```python
from build123d import *

# Parameters (mm, degrees)
SKETCH_2_R          = 32
EXTRUDE_2_DEPTH     = 1
SKETCH_3_R          = 32
EXTRUDE_3_DEPTH     = 28
EXTRUDE_3_TAPER     = 45
SKETCH_5_R          = 30
CUT_EXTRUDE_1_DEPTH = 1
SKETCH_6_R          = 30
CUT_EXTRUDE_2_DEPTH = 28
CUT_EXTRUDE_2_DRAFT = -45
SKETCH_7_R          = 4
EXTRUDE_5_DEPTH     = 6
EXTRUDE_5_TAPER     = 10
SKETCH_10_R         = 2
CUT_EXTRUDE_3_DEPTH = 54.749418721


with BuildPart() as part:
    # 草图2 → 凸台-拉伸2 (new body)
    with BuildSketch(Plane(origin=(0, 0, 0), x_dir=(1, 0, 0), z_dir=(0, 1, 0))):
        with Locations(Location((0, 0, 0), (0, 0, 270))):
            Circle(SKETCH_2_R)
    extrude(amount=EXTRUDE_2_DEPTH)

    # 草图3 → 凸台-拉伸3 (add)
    with BuildSketch(Plane(origin=(0, 1, 0), x_dir=(1, 0, 0), z_dir=(0, 1, 0))):
        with Locations(Location((0, 0, 0), (0, 0, 270))):
            Circle(SKETCH_3_R)
    extrude(amount=EXTRUDE_3_DEPTH, taper=EXTRUDE_3_TAPER)

    # 草图5 → 切除-拉伸1 (cut)
    with BuildSketch(Plane(origin=(0, 0, 0), x_dir=(-1, 0, 0), z_dir=(0, -1, 0))):
        with Locations(Location((0, 0, 0), (0, 0, 90))):
            Circle(SKETCH_5_R)
    extrude(amount=-CUT_EXTRUDE_1_DEPTH, mode=Mode.SUBTRACT)


with BuildPart() as cut_extrude_2_tool:
    # 草图6 → 切除-拉伸2 (with draft: the straight prism first)
    with BuildSketch(Plane(origin=(0, 1, 0), x_dir=(-1, 0, 0), z_dir=(0, -1, 0))):
        with Locations(Location((0, 0, 0), (0, 0, 90))):
            Circle(SKETCH_6_R)
    extrude(amount=-CUT_EXTRUDE_2_DEPTH)
    # 切除-拉伸2: the draft: its side faces are tilted about the plane it starts from
    cut_extrude_2_sides = [cut_extrude_2_tool.faces().sort_by_distance(p)[0] for p in [
        (0, 15, 30),
    ]]
    draft(cut_extrude_2_sides, Plane(origin=(0, 1, 0), x_dir=(-1, 0, 0), z_dir=(0, -1, 0)), CUT_EXTRUDE_2_DRAFT)


with BuildPart() as part_1:
    add(part.part)

    # 切除-拉伸2: cut by cut_extrude_2_tool
    add(cut_extrude_2_tool.part, mode=Mode.SUBTRACT)

    # 草图7 → 凸台-拉伸5 (add)
    with BuildSketch(Plane(origin=(0, 29, 0), x_dir=(1, 0, 0), z_dir=(0, 1, 0))):
        Circle(SKETCH_7_R)
    extrude(amount=EXTRUDE_5_DEPTH, taper=EXTRUDE_5_TAPER)

    # 草图10 → 切除-拉伸3 (cut, through all)
    with BuildSketch(Plane(origin=(0, 29, 0), x_dir=(-1, 0, 0), z_dir=(0, -1, 0))):
        with Locations(Location((0, 0, 0), (0, 0, 90))):
            Circle(SKETCH_10_R)
    extrude(amount=-CUT_EXTRUDE_3_DEPTH, mode=Mode.SUBTRACT)


solid = part_1.part
```
Design review of the part built by this model. Coordinates are the model's own, in mm. A direction names the side the tool comes from. Coordinates: 2 decimals unless noted, no trailing zeros. Order: outer loops, then holes, each group sorted by start corner. A loop starts at its lowest first (then second) coordinate and runs counter-clockwise, first axis right, second up. Notation, with made-up numbers: M 75.25,-37 L 119.25,-37 A20 ccw 119.25,-16 Z; hole C 56,80 d5. An arc over 180 degrees is marked long. Answer as a JSON object with one key per item and string values. Group by question number.
1) Mouldability with a two-part tool opening along Z and no side actions: class faces 3 (the conical face through (2.54, 24.53, 8.08)), 4 (the flat face through (1, 35, 2)), 5 (the conical face through (-6.699, 24.137, 1.488)) as pulls with the +Z half, pulls with the -Z half, needs draft (parallel to the pull), parting line crosses it, or undercut.
2) Tool access review of faces 1 (the cylindrical face through (1.32, 0.49, 29.97)), 2 (the conical face through (-0.436, 32.709, -3.318)): name each direction out of +Z, -Z, +X, -X, +Y, -Y from which nothing blocks a thin tool from reaching the whole face with its end or side.
3) Wall thickness on L1, parallel to X at y = 0.4, z = 0; L2, parallel to X at y = 5.5, z = -5 (3 decimals); L3, parallel to Z at x = -3.5, y = 17.5: over which ranges is each line inside the solid? List them lowest first.
4) Add section B-B, the plane y = 7.5. Write out the cut boundary in (x, z), then the cut area to 3 significant figures.
5) Add section A-A, the plane y = 20. Write out the cut boundary in (x, z).
6) For pin 1 (5 mm diameter, centred on x = 2.5, y = 18, fed in from +Z); pin 2 (3 mm diameter, centred on x = 7, y = 9, fed in from -Z); pin 3 (2 mm diameter, centred on x = 24, z = -9.5, fed in from -Y), all flat-tipped, find the tip position at first contact; note any pin that passes through.
Computed values:
{
 "1": {"face 3": "parting line crosses it", "face 4": "needs draft", "face 5": "undercut"},
 "2": {"face 1": "-Y", "face 2": "+Y"},
 "3": {"L1": "x = -32 to -30, 30 to 32", "L2": "x = -27.042 to -25.005, 25.005 to 27.042", "L3": "z = -15.1 to -13.04, 13.04 to 15.1"},
 "4": {"outline": "C 0,0 d51; hole C 0,0 d47", "area": "308 mm^2"},
 "5": {"outline": "C 0,0 d26; hole C 0,0 d22"},
 "6": {"pin 1": "stops at z = 17.34", "pin 2": "stops at z = -24.58", "pin 3": "stops at y = 4.19"}
}
